Can you work these out from the drawing? Everything is in mm from the part's minimum corner. A direction names the side the tool comes from. Round coordinates to 2 decimals unless told otherwise and drop trailing zeros. Write each loop counter-clockwise with the first axis right and the second up, starting at its lowest first coordinate (ties: lowest second). Pieces come first, ordered by that corner, then holes. Notation, with made-up numbers: M -6.75,74.25 L -0.75,74.25 A30 cw -0.75,96.25 Z; hole C 71,79 d6. An arc over 180 degrees is marked long. Use one line per item in the form item = value. Start each with the question number.
Q1. For the marked faces 1 and 2, which set-ups out of +Z, -Z, +X, -X, +Y, -Y let a thin tool reach every point of the face, with its end or its side?
Q2. I need wall thicknesses on line 1 along Y through (x, z) = (5.5, 9); line 2 along Y through (x, z) = (5, 26); line 3 along Z through (x, y) = (12, 32.5). Which ranges of each line are inside material? Lowest first, please. Write a range as from..to.
Q3. I'm going to push flat-ended pins straight in: pin 1 Ø4 at (x, y) = (36.5, 36.5) entering from +Z; pin 2 Ø1.8 at (x, y) = (5.5, 36.5) entering from -Z; pin 3 Ø4 at (x, y) = (10.5, 16) entering from +Z. Where does each tip first touch, or does it pass through?
Q4. I want a section at A-A on y = 5.5. List the corners of the cut face in (x, z) for me, and give its area (3 significant figures).
Q5. I want a section at B-B on z = 6.5. List the corners of the cut face in (x, y) for me.
Q6. I want a section at D-D on x = 21. List the corners of the cut face in (y, z) for me, and give its area (3 significant figures).
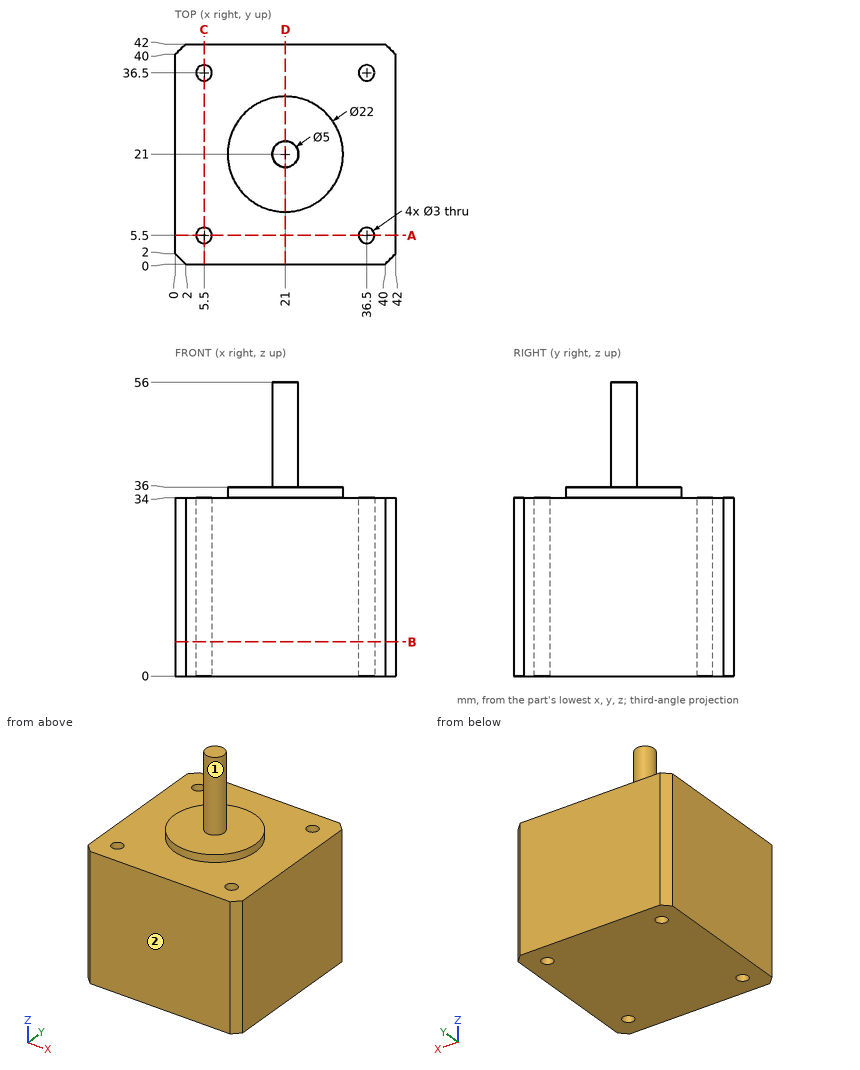
Reported:
q1.face_1 = +Z
q1.face_2 = +Z, -Z, +X, -X, -Y
q2.line_1 = 0..4, 7..35, 38..42
q2.line_2 = 0..4.09, 6.91..35.09, 37.91..42
q2.line_3 = 0..34
q3.pin_1 = 34
q3.pin_2 = through
q3.pin_3 = 36
q4.outline = M 0,0 L 4,0 L 4,34 L 0,34 Z; M 7,0 L 35,0 L 35,34 L 7,34 Z; M 38,0 L 42,0 L 42,34 L 38,34 Z
q4.area = 1,220 mm^2
q5.outline = M 0,2 L 2,0 L 40,0 L 42,2 L 42,40 L 40,42 L 2,42 L 0,40 Z; hole C 5.5,5.5 d3; hole C 5.5,36.5 d3; hole C 36.5,5.5 d3; hole C 36.5,36.5 d3
q6.outline = M 0,0 L 42,0 L 42,34 L 32,34 L 32,36 L 23.5,36 L 23.5,56 L 18.5,56 L 18.5,36 L 10,36 L 10,34 L 0,34 Z
q6.area = 1,570 mm^2
